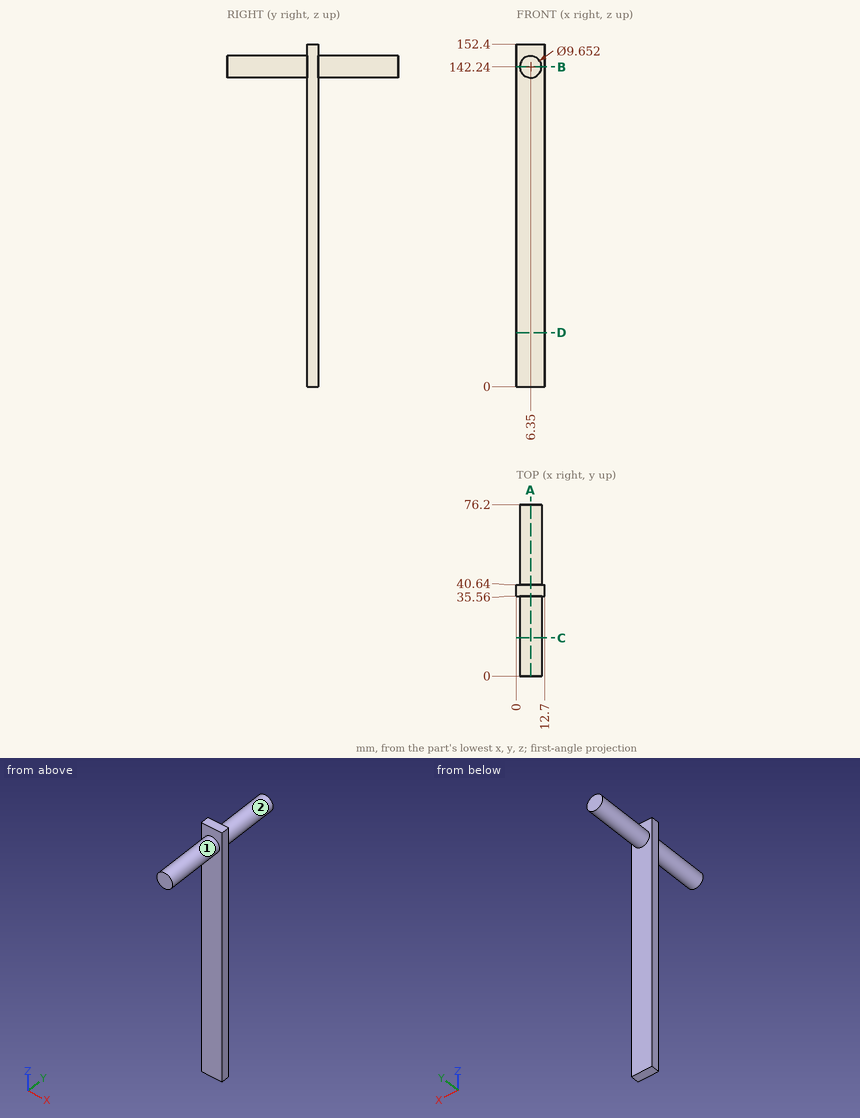
Study the drawing (mm; zero at the part's minimum x, y, z) and answer. A direction names the side the tool comes from. Give positions to 0.01 mm unless a question says otherwise; leave off trailing zeros. Order: outer loops, then holes, each group sorted by start corner. A loop starts at its lowest first (then second) coordinate and runs counter-clockwise, first axis right, second up. Notation, with made-up numbers: (53, 25) - (107, 25) arc R36 cw to (107, 60) - close; hole circle Ø6 at (26, -9). An arc over 180 degrees is marked (long way). Answer as CSV lines item,"result". Start each with the question number.
Q1. The part is cut by section A-A (x = 6.35). Write down the section's boundary in (y, z).
Q2. The part is cut by section B-B (z = 142.24). Write down the section's boundary in (x, y).
Q3. The part is cut by section D-D (z = 24). Write down the section's boundary in (x, y).
Q4. The part is cut by section C-C (y = 17). Write down the section's boundary in (x, z), then the cut area to 3 significant figures.
Q5. Find the intervals of material crossed by L1, parallel to Y at x = 11, z = 73.5; L2, parallel to Z at x = 5, y = 31; L3, parallel to Z at x = 2.75, y = 55, in increasing order. Write a range as [from, to].
Q6. For the marked faces 1 and 2, determine the directions among +Z, -Z, +X, -X, +Y, -Y from which every point of the face is accessible in a straight line to the end or side of a thin tool.
Q7. Given pin 1 Ø1 at (x, y) = (6.5, 50.5) entering from -Z; pin 2 Ø4 at (x, z) = (4, 97) entering from +Y; pin 3 Ø6.5 at (x, z) = (4.5, 70) entering from -Y, each flat-ended and moving along its own axis, determine where each tip first touches the part or whether it passes through.
Check result:
1,outline,"(0, 137.41) - (35.56, 137.41) - (35.56, 0) - (40.64, 0) - (40.64, 137.41) - (76.2, 137.41) - (76.2, 147.07) - (40.64, 147.07) - (40.64, 152.4) - (35.56, 152.4) - (35.56, 147.07) - (0, 147.07) - close"
2,outline,"(0, 35.56) - (1.52, 35.56) - (1.52, 0) - (11.18, 0) - (11.18, 35.56) - (12.7, 35.56) - (12.7, 40.64) - (11.18, 40.64) - (11.18, 76.2) - (1.52, 76.2) - (1.52, 40.64) - (0, 40.64) - close"
3,outline,"(0, 35.56) - (12.7, 35.56) - (12.7, 40.64) - (0, 40.64) - close"
4,outline,"circle Ø9.65 at (6.35, 142.24)"
4,area,"73.2 mm²"
5,L1,"y = [35.56, 40.64]"
5,L2,"z = [137.61, 146.87]"
5,L3,"z = [139.03, 145.45]"
6,face 1,"-Y"
6,face 2,"+Y"
7,pin 1,"stops at z = 137.41"
7,pin 2,"stops at y = 40.64"
7,pin 3,"stops at y = 35.56"
